Part model, mm, in its own coordinate system. Give positions to 0.01 mm unless a question says otherwise; leave off trailing zeros. Order: outer loops, then holes, each group sorted by start corner. A loop starts at its lowest first (then second) coordinate and runs counter-clockwise, first axis right, second up.
1. Probe line 1 (X direction, y = -23, z = 23.25); line 2 (Y direction, x = -60, z = 17); line 3 (Y direction, x = 100, z = 5). List the from-to ranges inside material, lowest first.
2. Slice it at A-A on y = 80. List the corners of the cut face in (x, z).
3. Drop flat-ended pins along their axis: pin 1 Ø1.5 at (x, y) = (176.5, 3.5) entering from +Z; pin 2 Ø5.5 at (y, z) = (-15, 20) entering from +X. Give the stop position or say it passes through.
from build123d import *

# Parameters (mm, degrees)
F0_W      = 350
F0_H      = 250
F1_DEPTH  = 25
F4_R      = 7.5
F4_R_2    = 5
F5_DEPTH  = 25.001
F10_W     = 5
F10_H     = 80
F11_DEPTH = 3
F12_W     = 13
F12_H     = 250
F13_DEPTH = 25
F14_W     = 3
F14_H     = 80
F15_DEPTH = 10
F16_R     = 3
F17_DEPTH = 10


with BuildPart() as f1:
    # F0 (on Top) → F1 (new body)
    with BuildSketch(Plane.XY):
        Rectangle(F0_W, F0_H)
    extrude(amount=F1_DEPTH)

    # F2 (on face) → F3 (revolve, cut)
    with BuildSketch(Plane.XY.offset(25)):
        Polygon((175, 0), (175, 0.25), (-125, 3), (-125, 0), align=None)
    revolve(axis=Axis((25, 0, 25), (1, 0, 0)), mode=Mode.SUBTRACT)

    # F4 (on face) → F5 (cut, through all)
    with BuildSketch(Plane.XY.offset(25)):
        with Locations((-60, 80)):
            Circle(F4_R)
        with Locations((-60, 80)):
            Circle(F4_R_2, mode=Mode.SUBTRACT)
        with Locations((-60, 80)):
            Circle(F4_R_2)
        with Locations((100, -80)):
            Circle(F4_R)
        with Locations((100, -80)):
            Circle(F4_R_2, mode=Mode.SUBTRACT)
        with Locations((100, -80)):
            Circle(F4_R_2)
    extrude(amount=-F5_DEPTH, mode=Mode.SUBTRACT)

    # F6 (on face) → F7 (revolve, cut)
    with BuildSketch(Plane.XY.offset(25)):
        Polygon((-125, 33), (-125, 30), (175, 30), (175, 30.5), align=None)
    revolve(axis=Axis((25, 30, 25), (1, 0, 0)), mode=Mode.SUBTRACT)

    # F8 (on face) → F9 (revolve, cut)
    with BuildSketch(Plane.XY.offset(25)):
        Polygon((175, -30), (-125, -30), (-125, -33), (175, -30.05), align=None)
    revolve(axis=Axis((25, -30, 25), (-1, 0, 0)), mode=Mode.SUBTRACT)

    # F10 (on face) → F11 (cut)
    with BuildSketch(Plane.XY.offset(25)):
        with Locations((-127.5, 0)):
            Rectangle(F10_W, F10_H)
        with BuildLine():
            Line((-130, 40), (-125, 40))
            ThreePointArc((-125, 40), (-127.5, 42.5), (-130, 40))
        make_face()
        with BuildLine():
            ThreePointArc((-130, -40), (-127.5, -42.5), (-125, -40))
            Line((-125, -40), (-130, -40))
        make_face()
    extrude(amount=-F11_DEPTH, mode=Mode.SUBTRACT)

    # F12 (on Top) → F13 (join)
    with BuildSketch(Plane.XY):
        with Locations((181.5, 0)):
            Rectangle(F12_W, F12_H)
    extrude(amount=F13_DEPTH)

    # F14 (on face) → F15 (cut)
    with BuildSketch(Plane.XY.offset(25)):
        with BuildLine():
            ThreePointArc((178, 40), (176.5, 41.5), (175, 40))
            Line((175, 40), (178, 40))
        make_face()
        with Locations((176.5, 0)):
            Rectangle(F14_W, F14_H)
        with BuildLine():
            Line((178, -40), (175, -40))
            ThreePointArc((175, -40), (176.5, -41.5), (178, -40))
        make_face()
    extrude(amount=-F15_DEPTH, mode=Mode.SUBTRACT)

    # F16 (on face) → F17 (cut, through all)
    with BuildSketch(Plane.YZ.offset(188)):
        with Locations((-15, 20)):
            Circle(F16_R)
    extrude(amount=-F17_DEPTH, mode=Mode.SUBTRACT)


solid = f1.part
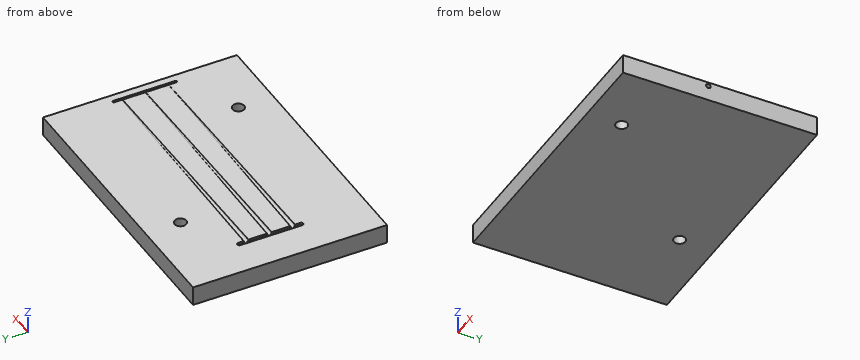
Data:
1. line 1: x = -175 to -130, -125 to 175, 178 to 188
1. line 2: y = -125 to 72.5, 87.5 to 125
1. line 3: y = -125 to -87.5, -72.5 to 125
2. outline: (-175, 0) - (-67.5, 0) - (-67.5, 25) - (-175, 25) - close; (-52.5, 0) - (188, 0) - (188, 25) - (-52.5, 25) - close
3. pin 1: stops at z = 15
3. pin 2: stops at x = 175
